```python
from build123d import *

# Parameters (mm, degrees)
F0_W     = 54.369731
F0_H     = 46.646759
F2_DEPTH = 254
F1_W     = 121.096216
F1_H     = 105.032436
F3_DEPTH = 1.27
F4_W     = 35.525674
F4_H     = 36.143513
F5_DEPTH = 127


with BuildPart() as f2:
    # F0 (on Top) → F2 (new body)
    with BuildSketch(Plane.XY):
        with Locations((-1.544595, -0.463377)):
            Rectangle(F0_W, F0_H)
    extrude(amount=-F2_DEPTH)

    # F1 (on Top) → F3 (join)
    with BuildSketch(Plane.XY):
        with Locations((2.78027, 1.235675)):
            Rectangle(F1_W, F1_H)
    extrude(amount=F3_DEPTH)

    # F4 (on face) → F5 (cut)
    with BuildSketch(Plane.XY.offset(1.27)):
        with Locations((1.699054, 5.40608)):
            Rectangle(F4_W, F4_H)
    extrude(amount=-F5_DEPTH, mode=Mode.SUBTRACT)


solid = f2.part
```
Model file for the job. Use its own axes, mm. A direction names the side the tool comes from. Coordinates: 2 decimals unless noted, no trailing zeros. Write each loop counter-clockwise with the first axis right and the second up, starting at its lowest first coordinate (ties: lowest second). Pieces come first, ordered by that corner, then holes. Notation, with made-up numbers: (24.5, 0.5) - (73.5, 0.5) arc R20 ccw to (73.5, 36.5) - close; hole circle Ø1 at (-17.5, -8.5). An arc over 180 degrees is marked (long way). One line per item, written item: value. Start each with the question number.
1. Slice it at D-D (x = 32). Write the cut outline in (y, z).
2. Flat gauge pins, fed straight in: pin 1 (4 mm diameter, centred on y = -20, z = -225, fed in from +X); pin 2 (1.5 mm diameter, centred on x = 31.5, y = 38, fed in from -Z); pin 3 (8 mm diameter, centred on x = 14.5, z = -183.5, fed in from +Y); pin 4 (4 mm diameter, centred on x = -29, y = 4, fed in from -Z). Where does each tip first touch, or does it go through?
3. Slice it at A-A (x = 17). Write the cut outline in (y, z).
4. Probe line 1 (X direction, y = 16, z = -79); line 2 (Z direction, x = 42.5, y = -12.5); line 3 (X direction, y = 11, z = -205). List the from-to ranges inside material, lowest first. Write a range as from..to.
5. Mould opens along X. For faces 5 (the flat face through (25.64, -1, -125)), 6 (the flat face through (2, -21, 1.27)), 7 (the flat face through (-16.064, 5, -61)) say: released by +X, released by -X, zero draft, split by the parting line, or undercut.
6. Slice it at C-C (z = -57.5). Write the cut outline in (x, y), plus the area to 3 significant figures.
7. Tool access for faces 1 (the flat face through (1, 5, -125.73)), 2 (the flat face through (-2, -23.787, -125)), 3 (the flat face through (-2, 22.86, -153)), 4 (the flat face through (-28.729, -1, -125)): list every direction of +Z, -Z, +X, -X, +Y, -Y with a clear straight run to the whole face (end or side of a thin tool).
8. Slice it at B-B (y = 0). Write the cut outline in (x, z), plus the area to 3 significant figures.
Answers below:
1. outline: (-51.28, 0) - (53.75, 0) - (53.75, 1.27) - (-51.28, 1.27) - close
2. pin 1: stops at x = 25.64
2. pin 2: stops at z = 0
2. pin 3: stops at y = 22.86
2. pin 4: stops at z = -254
3. outline: (-51.28, 0) - (-23.79, 0) - (-23.79, -254) - (22.86, -254) - (22.86, -125.73) - (-12.67, -125.73) - (-12.67, 1.27) - (-51.28, 1.27) - close; (23.48, 0) - (53.75, 0) - (53.75, 1.27) - (23.48, 1.27) - close
4. line 1: x = -28.73..-16.06, 19.46..25.64
4. line 2: z = 0..1.27
4. line 3: x = -28.73..25.64
5. face 5: released by +X
5. face 6: zero draft
5. face 7: undercut
6. outline: (-28.73, -23.79) - (25.64, -23.79) - (25.64, 22.86) - (19.46, 22.86) - (19.46, -12.67) - (-16.06, -12.67) - (-16.06, 22.86) - (-28.73, 22.86) - close
6. area: 1,270 mm^2
7. face 1: +Z, +Y
7. face 2: -Z, +X, -X, -Y
7. face 3: -Z, +X, -X, +Y
7. face 4: -Z, -X, +Y, -Y
8. outline: (-57.77, 0) - (-28.73, 0) - (-28.73, -254) - (25.64, -254) - (25.64, 0) - (63.33, 0) - (63.33, 1.27) - (19.46, 1.27) - (19.46, -125.73) - (-16.06, -125.73) - (-16.06, 1.27) - (-57.77, 1.27) - close
8. area: 9,450 mm^2
